from build123d import *

# Parameters (mm, degrees)
F0_R      = 1.75
F1_DEPTH  = 2
F2_DEPTH  = 25
F3_W      = 10
F3_H      = 11
F4_DEPTH  = 12.5
F5_W      = 16
F5_H      = 12
F5_W_2    = 9.587623179
F5_H_2    = 49.3407100439
F5_W_3    = 20
F5_H_3    = 3.5
F6_W      = 20
F6_H      = 4
F7_DEPTH  = 12.5
F8_R      = 3
F10_DEPTH = 7.5
F11_W     = 1
F11_H     = 42.6
F15_SIZE  = 2


# Not quite as in the source:
# - a feature names something its author has since deleted; it is built from what else it names


with BuildPart() as f1:
    # F0 (on Top) → F1 (new body)
    with BuildSketch(Plane.XY):
        Polygon((-15.5396774872, 50.4744988004), (-9.0115841546, 37.4744988004), (4.3894230769, 37.4744988004), (4.3894230769, 50.4744988004), align=None)
        with Locations((-9.6105769231, 47.4744988004)):
            Circle(F0_R, mode=Mode.SUBTRACT)
    extrude(amount=F1_DEPTH)



with BuildPart() as f1b:
    # F0 (on Top) → F1, piece 2 (new body)
    with BuildSketch(Plane.XY):
        Polygon((55.9884158454, 37.4744988004), (62.1997159179, 31.2), (67, 26.3508739936), (67, -26.3508739936), (62.1997159179, -31.2), (55.9884158454, -37.4744988004), (42.8894230769, -37.4744988004), (42.8894230769, -50.4744988004), (55.5480775622, -50.4744988004), (75, -30.8246569672), (75, 30.8246569672), (55.5480775622, 50.4744988004), (42.8894230769, 50.4744988004), (42.8894230769, 37.4744988004), align=None)
        with Locations((52.8894230769, -47.4744988004)):
            Circle(F0_R, mode=Mode.SUBTRACT)
        with Locations((69, -31.2)):
            Circle(F0_R, mode=Mode.SUBTRACT)
        with Locations((69, 31.2)):
            Circle(F0_R, mode=Mode.SUBTRACT)
        with Locations((52.8894230769, 47.4744988004)):
            Circle(F0_R, mode=Mode.SUBTRACT)
    extrude(amount=F1_DEPTH)


with BuildPart() as f1c:
    # F0 (on Top) → F1, piece 3 (new body)
    with BuildSketch(Plane.XY):
        Polygon((4.3894230769, -50.4744988004), (4.3894230769, -37.4744988004), (-9.0115841546, -37.4744988004), (-15.5396774872, -50.4744988004), align=None)
        with Locations((-9.6105769231, -47.4744988004)):
            Circle(F0_R, mode=Mode.SUBTRACT)
    extrude(amount=F1_DEPTH)


with BuildPart() as f1_1:
    add(f1.part)

    add(f1b.part)  # F2 merges F1b

    add(f1c.part)  # F2 merges F1c
    # F0 (on Top) → F2 (join)
    with BuildSketch(Plane.XY):
        with BuildLine():
            ThreePointArc((-1, 31.2), (2, 34.2), (5, 31.2))
            Line((5, 31.2), (38.7, 31.2))
            ThreePointArc((38.7, 31.2), (41.7, 34.2), (44.7, 31.2))
            Line((44.7, 31.2), (54.1997159179, 31.2))
            Line((54.1997159179, 31.2), (62.1997159179, 31.2))
            Line((62.1997159179, 31.2), (55.9884158454, 37.4744988004))
            Line((55.9884158454, 37.4744988004), (42.8894230769, 37.4744988004))
            Line((42.8894230769, 37.4744988004), (4.3894230769, 37.4744988004))
            Line((4.3894230769, 37.4744988004), (-9.0115841546, 37.4744988004))
            Line((-9.0115841546, 37.4744988004), (-5.9652768733, 31.4081035087))
            Line((-5.9652768733, 31.4081035087), (-5.8607754019, 31.2))
            Line((-5.8607754019, 31.2), (-1, 31.2))
        make_face()
        with BuildLine():
            Line((55.9884158454, -37.4744988004), (62.1997159179, -31.2))
            Line((62.1997159179, -31.2), (54.1997159179, -31.2))
            Line((54.1997159179, -31.2), (44.7, -31.2))
            ThreePointArc((44.7, -31.2), (41.7, -34.2), (38.7, -31.2))
            Line((38.7, -31.2), (5, -31.2))
            ThreePointArc((5, -31.2), (2, -34.2), (-1, -31.2))
            Line((-1, -31.2), (-5.8607754019, -31.2))
            Line((-5.8607754019, -31.2), (-5.9652768733, -31.4081035087))
            Line((-5.9652768733, -31.4081035087), (-9.0115841546, -37.4744988004))
            Line((-9.0115841546, -37.4744988004), (4.3894230769, -37.4744988004))
            Line((4.3894230769, -37.4744988004), (42.8894230769, -37.4744988004))
            Line((42.8894230769, -37.4744988004), (55.9884158454, -37.4744988004))
        make_face()
        Polygon((62.1997159179, 31.2), (54.1997159179, 31.2), (59.0998579589, 26.25), (64, 21.3), (64, -21.3), (59.0998579589, -26.25), (54.1997159179, -31.2), (62.1997159179, -31.2), (67, -26.3508739936), (67, 26.3508739936), align=None)
        with BuildLine():
            Line((38.7, 31.2), (5, 31.2))
            ThreePointArc((5, 31.2), (2, 28.2), (-1, 31.2))
            Line((-1, 31.2), (-5.8607754019, 31.2))
            Line((-5.8607754019, 31.2), (-3.3750783253, 26.25))
            Line((-3.3750783253, 26.25), (59.0998579589, 26.25))
            Line((59.0998579589, 26.25), (54.1997159179, 31.2))
            Line((54.1997159179, 31.2), (44.7, 31.2))
            ThreePointArc((44.7, 31.2), (41.7, 28.2), (38.7, 31.2))
        make_face()
        with BuildLine():
            Line((54.1997159179, -31.2), (59.0998579589, -26.25))
            Line((59.0998579589, -26.25), (-3.3750783253, -26.25))
            Line((-3.3750783253, -26.25), (-5.8607754019, -31.2))
            Line((-5.8607754019, -31.2), (-1, -31.2))
            ThreePointArc((-1, -31.2), (2, -28.2), (5, -31.2))
            Line((5, -31.2), (38.7, -31.2))
            ThreePointArc((38.7, -31.2), (41.7, -28.2), (44.7, -31.2))
            Line((44.7, -31.2), (54.1997159179, -31.2))
        make_face()
    extrude(amount=F2_DEPTH)

    # F3 (on face) → F4 (cut, symmetric)
    with BuildSketch(Plane.YZ.offset(67)):
        with Locations((-5, 15.5)):
            Rectangle(F3_W, F3_H)
        with Locations((5, 15.5)):
            Rectangle(F3_W, F3_H)
    extrude(amount=F4_DEPTH, both=True, mode=Mode.SUBTRACT)

    # F5 (on face) + F6 (on face) → F7 (cut, symmetric)
    with BuildSketch(Plane.XZ.offset(37.4744988004)):
        with Locations((31.4884158454, 13.5)):
            Rectangle(F5_W, F5_H)
        with Locations((88.4978957474, 268.2395651937)):
            Rectangle(F5_W_2, F5_H_2)
        with Locations((25.8894230769, 1.75)):
            Rectangle(F5_W_3, F5_H_3)
    with BuildSketch(Plane(origin=(0, 37.4744988004, 0), x_dir=(-1, 0, 0), z_dir=(0, 1, 0))):
        with Locations((-22.8894230769, 2)):
            Rectangle(F6_W, F6_H)
    extrude(amount=F7_DEPTH, both=True, dir=(0, -1, 0), mode=Mode.SUBTRACT)

    # F8
    f8_edges = [f1_1.edges().sort_by_distance(p)[0] for p in [
        (49.438919, 37.474499, 2),
        (-2.311081, 37.474499, 2),
        (61.494208, 31.912686, 2),
        (67, 0, 2),
        (61.494208, -31.912686, 2),
        (49.438919, -37.474499, 2),
        (-2.311081, -37.474499, 2),
        (4.389423, 37.474499, 1),
        (42.889423, 37.474499, 1),
        (4.389423, -37.474499, 1),
        (42.889423, -37.474499, 1),
        (-15.539677, 50.474499, 1),
        (-15.539677, -50.474499, 1),
        (42.889423, 50.474499, 1),
        (4.389423, 50.474499, 1),
        (42.889423, -50.474499, 1),
        (4.389423, -50.474499, 1),
    ]]
    fillet(f8_edges, radius=F8_R)

    # F9 (on face) → F10 (cut)
    with BuildSketch(Plane(origin=(0, 0, 0), x_dir=(1, 0, 0), z_dir=(0, 0, -1))):
        with BuildLine():
            ThreePointArc((51.35, 31.2), (55.35, 27.2), (59.35, 31.2))
            ThreePointArc((59.35, 31.2), (55.35, 35.2), (51.35, 31.2))
        make_face()
        with BuildLine():
            Line((59.35, 26.25), (59.35, 31.2))
            ThreePointArc((59.35, 31.2), (55.35, 27.2), (51.35, 31.2))
            Line((51.35, 31.2), (51.35, 26.25))
            Line((51.35, 26.25), (59.0998579589, 26.25))
            Line((59.0998579589, 26.25), (59.35, 26.25))
        make_face()
        Polygon((59.35, 25.997312814), (59.35, 26.25), (59.0998579589, 26.25), align=None)
        with BuildLine():
            ThreePointArc((51.35, -31.2), (55.35, -35.2), (59.35, -31.2))
            ThreePointArc((59.35, -31.2), (55.35, -27.2), (51.35, -31.2))
        make_face()
        with BuildLine():
            ThreePointArc((51.35, -31.2), (55.35, -27.2), (59.35, -31.2))
            Line((59.35, -31.2), (59.35, -26.25))
            Line((59.35, -26.25), (59.0998579589, -26.25))
            Line((59.0998579589, -26.25), (51.35, -26.25))
            Line((51.35, -26.25), (51.35, -31.2))
        make_face()
        Polygon((59.0998579589, -26.25), (59.35, -26.25), (59.35, -25.997312814), align=None)
    extrude(amount=-F10_DEPTH, mode=Mode.SUBTRACT)

    # F11 (on face) → F12 (revolve, cut)
    with BuildSketch(Plane.XY.offset(25)):
        with Locations((66, 0)):
            Rectangle(F11_W, F11_H)
    revolve(axis=Axis((65.5, 0, 25), (0, -1, 0)), mode=Mode.SUBTRACT)

    # F11 (on face) → F13 (revolve, cut)
    with BuildSketch(Plane.XY.offset(25)):
        with BuildLine():
            ThreePointArc((3.9843134833, 33.45), (4.7343134833, 32.4343134833), (5, 31.2))
            Line((5, 31.2), (38.7, 31.2))
            ThreePointArc((38.7, 31.2), (38.9656865167, 32.4343134833), (39.7156865167, 33.45))
            Line((39.7156865167, 33.45), (3.9843134833, 33.45))
        make_face()
    revolve(axis=Axis((21.85, 31.2, 25), (1, 0, 0)), mode=Mode.SUBTRACT)

    # F11 (on face) → F14 (revolve, cut)
    with BuildSketch(Plane.XY.offset(25)):
        with BuildLine():
            Line((5, -31.2), (38.7, -31.2))
            ThreePointArc((38.7, -31.2), (38.9656865167, -29.9656865167), (39.7156865167, -28.95))
            Line((39.7156865167, -28.95), (3.9843134833, -28.95))
            ThreePointArc((3.9843134833, -28.95), (4.7343134833, -29.9656865167), (5, -31.2))
        make_face()
    revolve(axis=Axis((21.85, -31.2, 25), (1, 0, 0)), mode=Mode.SUBTRACT)

    # F15
    f15_edges = [f1_1.edges().sort_by_distance(p)[0] for p in [
        (65.5, -10, 21),
        (65.5, 10, 21),
        (65.5, -10, 10),
        (65.5, 10, 10),
    ]]
    chamfer(f15_edges, length=F15_SIZE)


solid = f1_1.part
The model under review builds one solid part; all positions refer to its coordinate system, in mm. A direction names the side the tool comes from. Give positions to 0.01 mm unless a question says otherwise; leave off trailing zeros. Order: outer loops, then holes, each group sorted by start corner. A loop starts at its lowest first (then second) coordinate and runs counter-clockwise, first axis right, second up. Notation, with made-up numbers: M -1.5,65 L 26.5,65 A27 cw 26.5,86 Z; hole C -29.5,87 d5. An arc over 180 degrees is marked long. Answer in a Markdown table with one row per item. Add a question column.
1. Add section B-B on y = 6.5. State the section outline as (x, z) points, plus the area to 3 significant figures.
2. For pin 1 Ø0.9 at (x, z) = (65, 14) entering from -Y; pin 2 Ø5.5 at (y, z) = (29.5, 2.5) entering from -X; pin 3 Ø3 at (y, z) = (26, 6) entering from -X, all flat-tipped, find the tip position at first contact; note any pin that passes through.
3. Add section D-D on y = -12. State the section outline as (x, z) points.
4. Add section C-C on x = 41.7. State the section outline as (y, z) points, plus the area to 3 significant figures.
5. Mouldability with a two-part tool opening along X and no side actions: class faces 1 (the cylindrical face through (-13.252, -49.013, 1.014)), 2 (the cylindrical face through (-7.994, 46.804, 0.986)), 3 (the flat face through (21, -26.25, 12)) as released by +X, released by -X, zero draft, split by the parting line, or undercut.
6. Add section A-A on z = 13.25. State the section outline as (x, y) points, plus the area to 3 significant figures.
7. Machinability: for faces 4 (the flat face through (55, 31, 7.5)), 5 (the flat face through (66, 10, 15)), 6 (the flat face through (71, 0, 2)), 7 (the cylindrical face through (43.74, -49.57, 1.01)), which of the approach directions +Z, -Z, +X, -X, +Y, -Y give a long, thin tool a straight path to every point of the face, cutting with its end or side? Answer none if there is none.
8. To check wall thickness, follow line 1 along X through (y, z) = (31.2, 12.75); line 2 along Y through (x, z) = (41.7, 9); line 3 along Y through (x, z) = (33, 5.75). State the ranges of each line that lie inside material, in increasing order.
The answers:
| question | item | result |
|---|---|---|
| 1 | outline | M 64,0 L 75,0 L 75,2 L 70,2 A3 cw 67,5 L 67,10 L 64,10 Z; M 64,21 L 67,21 L 67,25 L 66.5,25 A1 cw 64.5,25 L 64,25 Z |
| 1 | area | 58.4 mm2 |
| 2 | pin 1 | y = -28.83 |
| 2 | pin 2 | x = -6.39 |
| 2 | pin 3 | x = -4 |
| 3 | outline | M 64,0 L 75,0 L 75,2 L 70,2 A3 cw 67,5 L 67,25 L 66.5,25 A1 cw 64.5,25 L 64,25 Z |
| 4 | outline | M -38.08,0 L -34.2,0 L -34.2,25 L -37.47,25 L -37.47,5 A3 cw -38.08,3.19 Z; M -28.2,0 L -26.25,0 L -26.25,25 L -28.2,25 Z; M 26.25,0 L 28.2,0 L 28.2,25 L 26.25,25 Z; M 34.2,0 L 38.08,0 L 38.08,3.19 A3 cw 37.47,5 L 37.47,25 L 34.2,25 Z |
| 4 | area | 266 mm2 |
| 5 | face 1 | released by -X |
| 5 | face 2 | undercut |
| 5 | face 3 | zero draft |
| 6 | outline | M -9.01,-37.47 L 23.49,-37.47 L 23.49,-26.25 L -3.38,-26.25 Z; M -9.01,37.47 L -3.38,26.25 L 59.1,26.25 L 64,21.3 L 64,10 L 67,10 L 67,26.35 L 55.99,37.47 Z; M 39.49,-37.47 L 55.99,-37.47 L 67,-26.35 L 67,-10 L 64,-10 L 64,-21.3 L 59.1,-26.25 L 39.49,-26.25 L 39.49,-29.17 A3 cw long 39.49,-33.23 Z; hole C 2,-31.2 d6; hole C 2,31.2 d6; hole C 41.7,31.2 d6 |
| 6 | area | 1,350 mm2 |
| 7 | face 4 | -Z |
| 7 | face 5 | +X, -X |
| 7 | face 6 | +Z, +X |
| 7 | face 7 | +Z, -Z, -Y |
| 8 | line 1 | -5.86 to -1, 5 to 38.7, 44.7 to 62.2 |
| 8 | line 2 | -37.47 to -34.2, -28.2 to -26.25, 26.25 to 28.2, 34.2 to 37.47 |
| 8 | line 3 | -37.47 to -26.25, 26.25 to 37.47 |
